For this review, take the finished solid that the model builds, in its own axes (mm). A direction names the side the tool comes from. Round coordinates to 2 decimals unless told otherwise and drop trailing zeros. Write each loop counter-clockwise with the first axis right and the second up, starting at its lowest first coordinate (ties: lowest second). Pieces come first, ordered by that corner, then holes. Notation, with made-up numbers: (23, -11.5) -> (65, -11.5) arc R28 cw to (65, 23.5) -> close; hole circle Ø10 at (-3.75, 2). An arc over 180 degrees is marked (long way). Write each question's results on one line, items separated by ' | '. Start each with the question number.
Item 1: Tool access review of faces 1 (the flat face through (24, -9, -3)), 2 (the flat face through (-18.5, -11.8, -3.1)), 3 (the flat face through (-27, -13, -3)), 4 (the cylindrical face through (-20.206, 13.848, -1.726)), 5 (the flat face through (-8, 14, 0)): name each direction out of +Z, -Z, +X, -X, +Y, -Y from which nothing blocks a thin tool from reaching the whole face with its end or side.
Item 2: Add section D-D (x = -15). State the section outline as (y, z) points, plus the area to 4 significant figures.
Item 3: Clearance check with flat-ended pins moving along their axes: pin 1 (1.8 mm diameter, centred on x = 21.5, y = -15.5, fed in from +Z); pin 2 (1.9 mm diameter, centred on x = -21.59, y = -16.51, fed in from -Z); pin 3 (2 mm diameter, centred on y = 4, z = -4.5, fed in from +X). State where each tip first meets the part, or that it passes through.
Item 4: Add section A-A (x = -21.59). State the section outline as (y, z) points.
Item 5: The part is to be moulded in two halves that separate along Y. For faces 6 (the flat face through (0, 20.3, -3)), 7 (the cylindrical face through (-20.41, 17.59, -4.94)), 8 (the flat face through (-2, 14, -6.35)), say which applies: +Y half, -Y half, draft (parallel to the pull), parting line (faces both ways), or undercut.
Item 6: Add section C-C (y = 16.51). State the section outline as (x, z) points.
Item 7: Add section B-B (z = -1.75). State the section outline as (x, y) points, plus the area to 3 significant figures.
Item 8: To check wall thickness, follow line 1 along Y through (x, z) = (21.59, -4.65); line 2 along Y through (x, z) = (21.5, -1); line 3 along Y through (x, z) = (-21.59, -2.4). State the ranges of each line that lie inside material, in increasing order.
from build123d import *

# Parameters (mm, degrees)
F1_DEPTH       = 6.35
F2_D           = 3.2
F2_CBORE_D     = 6
F2_CBORE_DEPTH = 3.5
F3_SIZE        = 1


with BuildPart() as f1:
    # F0 (on Top) → F1 (new body)
    with BuildSketch(Plane.XY):
        Polygon((-27, -20.3), (27, -20.3), (27, -9), (21, -9), (21, -9.8), (16, -13.8), (-16, -13.8), (-21, -9.8), (-21, 9.8), (-16, 13.8), (16, 13.8), (21, 9.8), (21, 9), (27, 9), (27, 20.3), (-27, 20.3), (-27, 6.5), (-30, 3.5), (-30, -3.5), (-27, -6.5), align=None)
    extrude(amount=-F1_DEPTH)

    # F2 (through all)
    with Locations(Plane.XY):
        with Locations((-21.59, -16.51), (21.59, -16.51), (21.59, 16.51), (-21.59, 16.51)):
            CounterBoreHole(F2_D / 2, F2_CBORE_D / 2, F2_CBORE_DEPTH)

    # F3
    f3_edges = [f1.edges().sort_by_distance(p)[0] for p in [
        (-30, 0, 0),
    ]]
    chamfer(f3_edges, length=F3_SIZE)


solid = f1.part
Responses:
1) face 1: +Z, -Z, +X | face 2: +Z, -Z | face 3: +Z, -Z, -X, -Y | face 4: +Z | face 5: +Z, +X, -X, +Y, -Y
2) outline: (-20.3, -6.35) -> (-13.8, -6.35) -> (-13.8, 0) -> (-20.3, 0) -> close; (13.8, -6.35) -> (20.3, -6.35) -> (20.3, 0) -> (13.8, 0) -> close | area: 82.55 mm^2
3) pin 1: stops at z = -3.5 | pin 2: passes through | pin 3: stops at x = -21
4) outline: (-20.3, -6.35) -> (-18.11, -6.35) -> (-18.11, -3.5) -> (-19.51, -3.5) -> (-19.51, 0) -> (-20.3, 0) -> close; (-14.91, -6.35) -> (14.91, -6.35) -> (14.91, -3.5) -> (13.51, -3.5) -> (13.51, 0) -> (-13.51, 0) -> (-13.51, -3.5) -> (-14.91, -3.5) -> close; (18.11, -6.35) -> (20.3, -6.35) -> (20.3, 0) -> (19.51, 0) -> (19.51, -3.5) -> (18.11, -3.5) -> close
5) face 6: +Y half | face 7: undercut | face 8: draft
6) outline: (-27, -6.35) -> (-23.19, -6.35) -> (-23.19, -3.5) -> (-24.59, -3.5) -> (-24.59, 0) -> (-27, 0) -> close; (-19.99, -6.35) -> (19.99, -6.35) -> (19.99, -3.5) -> (18.59, -3.5) -> (18.59, 0) -> (-18.59, 0) -> (-18.59, -3.5) -> (-19.99, -3.5) -> close; (23.19, -6.35) -> (27, -6.35) -> (27, 0) -> (24.59, 0) -> (24.59, -3.5) -> (23.19, -3.5) -> close
7) outline: (-30, -3.5) -> (-27, -6.5) -> (-27, -20.3) -> (27, -20.3) -> (27, -9) -> (21, -9) -> (21, -9.8) -> (16, -13.8) -> (-16, -13.8) -> (-21, -9.8) -> (-21, 9.8) -> (-16, 13.8) -> (16, 13.8) -> (21, 9.8) -> (21, 9) -> (27, 9) -> (27, 20.3) -> (-27, 20.3) -> (-27, 6.5) -> (-30, 3.5) -> close; hole circle Ø6 at (-21.59, -16.51); hole circle Ø6 at (-21.59, 16.51); hole circle Ø6 at (21.59, -16.51); hole circle Ø6 at (21.59, 16.51) | area: 882 mm^2
8) line 1: y = -20.3 to -18.11, -14.91 to -9, 9 to 14.91, 18.11 to 20.3 | line 2: y = -20.3 to -19.51, -13.51 to -9, 9 to 13.51, 19.51 to 20.3 | line 3: y = -20.3 to -19.51, -13.51 to 13.51, 19.51 to 20.3
